```python
from build123d import *

# Parameters (mm, degrees)
F0_W     = 49.5728366077
F0_H     = 49.0062981844
F1_DEPTH = 79.9
F2_W     = 49.5728366077
F2_H     = 8.2149282098
F3_DEPTH = 45
F4_R     = 10
F5_R     = 5


with BuildPart() as f1:
    # F0 (on Front) → F1 (new body)
    with BuildSketch(Plane.XZ):
        Rectangle(F0_W, F0_H)
    extrude(amount=-F1_DEPTH)

    # F2 (on face) → F3 (join)
    with BuildSketch(Plane(origin=(0, 79.9, 0), x_dir=(-1, 0, 0), z_dir=(0, 1, 0))):
        with Locations((0, -20.3956849873)):
            Rectangle(F2_W, F2_H)
    extrude(amount=F3_DEPTH)

    # F4
    f4_edges = [f1.edges().sort_by_distance(p)[0] for p in [
        (0, 0, 24.503149),
    ]]
    fillet(f4_edges, radius=F4_R)

    # F5
    f5_edges = [f1.edges().sort_by_distance(p)[0] for p in [
        (24.786418, 2.928932, 21.574217),
        (-24.786418, 2.928932, 21.574217),
    ]]
    fillet(f5_edges, radius=F5_R)


solid = f1.part
```
Check sheet for the modelled part. Datum: model origin and axes. Units: mm. A direction names the side the tool comes from. Round coordinates to 2 decimals unless told otherwise and drop trailing zeros. Order: outer loops, then holes, each group sorted by start corner. A loop starts at its lowest first (then second) coordinate and runs counter-clockwise, first axis right, second up. Notation, with made-up numbers: (87.25, 27) - (144.25, 27) arc R24 cw to (144.25, 41) - close; hole circle Ø5 at (-13, -18). An arc over 180 degrees is marked (long way). Answer as CSV lines item,"result". Start each with the question number.
1) Tool access check on faces 1 (the face through (0.277, 2.852, 21.496)), 2 (the face through (0, 102, -16.288)). Record the directions out of +Z, -Z, +X, -X, +Y, -Y that give a thin tool (end or side, any length) a straight path to the whole face; none if there is none.
2) Section check C-C (y = 109.5). Record the cut outline in (x, z).
3) Section check A-A (x = -6). Record the cut outline in (y, z).
4) Scan lines: probe 1 along Z at (x, y) = (18.5, 97); probe 2 along Y at (x, z) = (-6, -3.5); probe 3 along Y at (x, z) = (6, 21). Record each from-to range of solid material in increasing order.
5) Depth check by flat-ended pin: pin 1 (12 mm diameter, centred on x = 4.5, z = 8.5, fed in from +Y); pin 2 (22.5 mm diameter, centred on x = 1.5, y = 96, fed in from +Z). Enter the tip coordinate at first touch or a pass-through.
6) Section check B-B (z = 10). Record the cut outline in (x, y).
Determined:
1,face 1,"+Z, +X, -X, -Y"
1,face 2,"+Z, +X, -X, +Y"
2,outline,"(-24.79, -24.5) - (24.79, -24.5) - (24.79, -16.29) - (-24.79, -16.29) - close"
3,outline,"(0, -24.5) - (124.9, -24.5) - (124.9, -16.29) - (79.9, -16.29) - (79.9, 24.5) - (10, 24.5) arc R10 ccw to (0, 14.5) - close"
4,probe 1,"-24.5 to -16.29"
4,probe 2,"0 to 79.9"
4,probe 3,"2.4 to 79.9"
5,pin 1,"y = 79.9"
5,pin 2,"z = -16.29"
6,outline,"(-24.79, 5) arc R5 ccw to (-19.79, 0) - (19.79, 0) arc R5 ccw to (24.79, 5) - (24.79, 79.9) - (-24.79, 79.9) - close"
